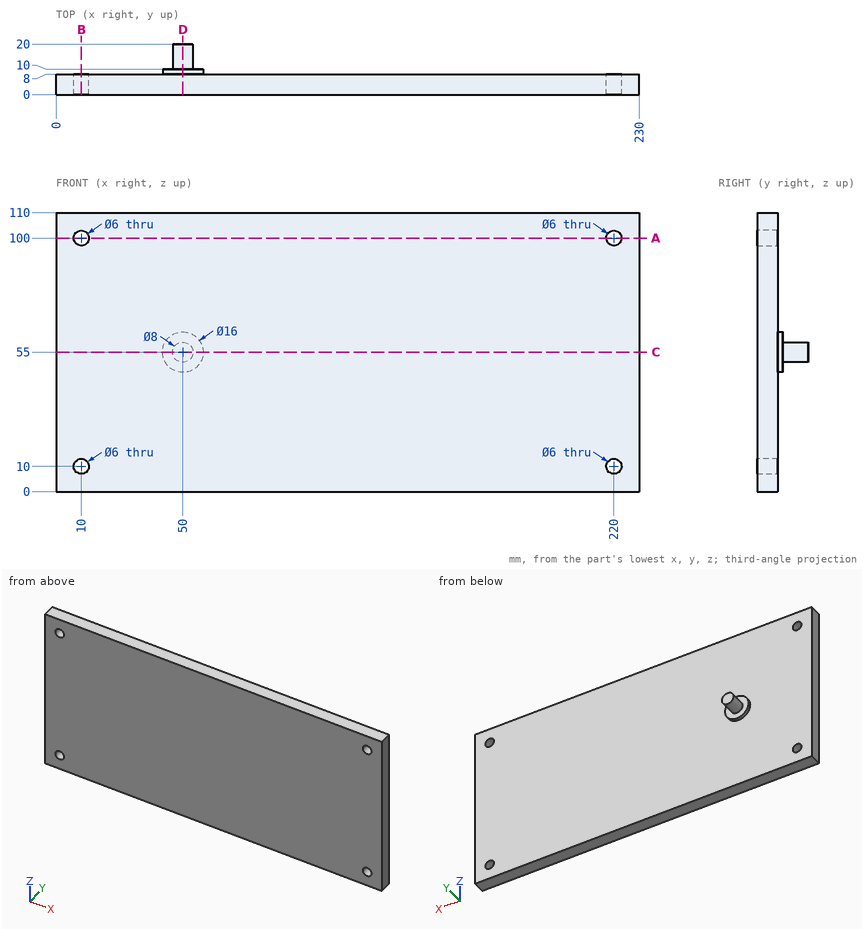
Geometry: see drawing. Coordinates: mm, zero at the bounding-box minimum. Round coordinates to 2 decimals unless told otherwise and drop trailing zeros. Write each loop counter-clockwise with the first axis right and the second up, starting at its lowest first coordinate (ties: lowest second). Pieces come first, ordered by that corner, then holes.
Item 1: Material intervals for L1, parallel to Z at x = 220, y = 2.5; L2, parallel to X at y = 4.25, z = 10; L3, parallel to Y at x = 122.5, z = 39.5, sorted ascending.
Item 2: Section query B-B (x = 10). Return loops of the section in (y, z), plus the area to 3 significant figures.
Item 3: Pin query (flat end, axial travel): P1, Ø2, axis at x = 80, z = 18.5, coming from the +Y side; P2, Ø1, axis at x = 42.5, y = 9.5, coming from the +Z side. Return the tip coordinate at first contact, or that it passes through.
Item 4: Section query A-A (z = 100). Return loops of the section in (x, y), plus the area to 3 significant figures.
Item 5: Section query C-C (z = 55). Return loops of the section in (x, y), plus the area to 3 significant figures.
Item 6: Section query D-D (x = 50). Return loops of the section in (y, z).
Completed:
1. L1: z = 0 to 7, 13 to 97, 103 to 110
1. L2: x = 0 to 7, 13 to 217, 223 to 230
1. L3: y = 0 to 8
2. outline: (0, 0) - (8, 0) - (8, 7) - (0, 7) - close; (0, 13) - (8, 13) - (8, 97) - (0, 97) - close; (0, 103) - (8, 103) - (8, 110) - (0, 110) - close
2. area: 784 mm2
3. P1: stops at y = 8
3. P2: stops at z = 58.87
4. outline: (0, 0) - (7, 0) - (7, 8) - (0, 8) - close; (13, 0) - (217, 0) - (217, 8) - (13, 8) - close; (223, 0) - (230, 0) - (230, 8) - (223, 8) - close
4. area: 1,740 mm2
5. outline: (0, 0) - (230, 0) - (230, 8) - (58, 8) - (58, 10) - (54, 10) - (54, 20) - (46, 20) - (46, 10) - (42, 10) - (42, 8) - (0, 8) - close
5. area: 1,950 mm2
6. outline: (0, 0) - (8, 0) - (8, 47) - (10, 47) - (10, 51) - (20, 51) - (20, 59) - (10, 59) - (10, 63) - (8, 63) - (8, 110) - (0, 110) - close
